The figure shows three views and two pictorial views of one solid part (mm, origin at its lowest corner). Answer the questions. A direction names the side the tool comes from. Coordinates: 2 decimals unless noted, no trailing zeros. Loops run counter-clockwise (first coordinate to the right, second up) from the corner with the lowest first, then second, coordinate; pieces in that order, holes last.
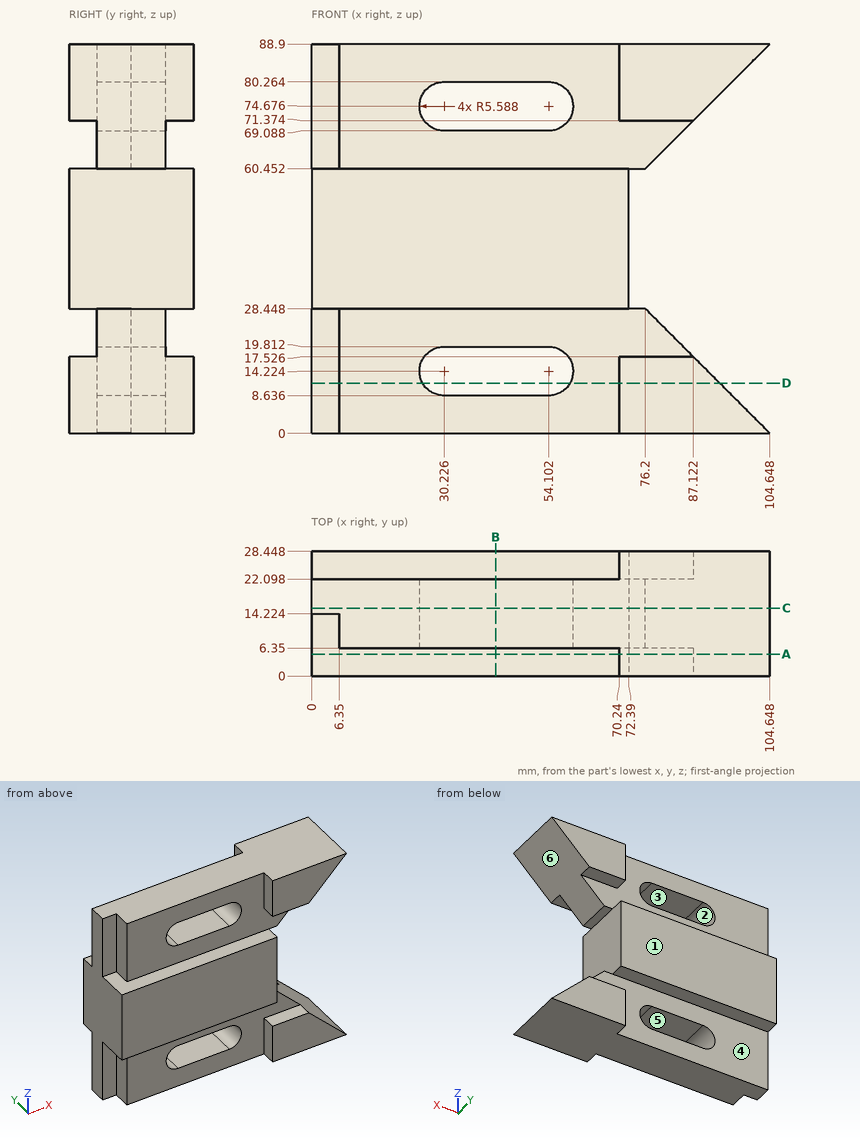
1. A cutting plane is placed at D-D, the plane z = 11.5. Give the vertices of the cut face in (x, y), then the cut area to 3 significant figures.
2. For the marked faces 1 and 2, determine the directions among +Z, -Z, +X, -X, +Y, -Y from which every point of the face is accessible in a straight line to the end or side of a thin tool.
3. A cutting plane is placed at C-C, the plane y = 15.5. Give the vertices of the cut face in (x, z), then the cut area to 3 significant figures.
4. A cutting plane is placed at B-B, the plane x = 42. Give the vertices of the cut face in (y, z), then the cut area to 3 significant figures.
5. Straight lines are drawn through the part: probe 1 along Z at (x, y) = (44.5, 6.75); probe 2 along Z at (x, y) = (78.5, 3.75); probe 3 along Y at (x, z) = (23.5, 19.5). For each, find the intervals that lie inside material, in ascending order.
6. Determine the mould class of the marked faces 3, 4, 5 and 6 for opening direction X: released by +X, released by -X, zero draft, split by the parting line, or undercut.
7. A cutting plane is placed at A-A, the plane y = 5. Give the vertices of the cut face in (x, z).
8. Each of these flat-tipped pins is pushed along its axis until it touches: P1, Ø3, axis at x = 27, y = 26, coming from the -Z side; P2, Ø3, axis at x = 3, z = 75.5, coming from the -Y side; P3, Ø5, axis at x = 23, z = 72, coming from the +Y side; P4, Ø8.5, axis at x = 43.5, z = 15, coming from the +Y side. Where does it stop, or does it pass through?
Answers below:
1. outline: (0, 14.22) - (6.35, 14.22) - (6.35, 6.35) - (25.35, 6.35) - (25.35, 22.1) - (0, 22.1) - close; (58.98, 6.35) - (70.24, 6.35) - (70.24, 0) - (93.15, 0) - (93.15, 28.45) - (70.24, 28.45) - (70.24, 22.1) - (58.98, 22.1) - close
1. area: 1,180 mm2
2. face 1: +Z, -Z, +X, -X, +Y
2. face 2: +Y, -Y
3. outline: (0, 0) - (104.65, 0) - (76.2, 28.45) - (72.39, 28.45) - (72.39, 60.45) - (76.2, 60.45) - (104.65, 88.9) - (0, 88.9) - close; hole (30.23, 8.64) - (54.1, 8.64) arc R5.59 ccw to (54.1, 19.81) - (30.23, 19.81) arc R5.59 ccw to start; hole (30.23, 69.09) - (54.1, 69.09) arc R5.59 ccw to (54.1, 80.26) - (30.23, 80.26) arc R5.59 ccw to start
3. area: 6,730 mm2
4. outline: (0, 28.45) - (6.35, 28.45) - (6.35, 19.81) - (22.1, 19.81) - (22.1, 28.45) - (28.45, 28.45) - (28.45, 60.45) - (22.1, 60.45) - (22.1, 69.09) - (6.35, 69.09) - (6.35, 60.45) - (0, 60.45) - close; (6.35, 0) - (22.1, 0) - (22.1, 8.64) - (6.35, 8.64) - close; (6.35, 80.26) - (22.1, 80.26) - (22.1, 88.9) - (6.35, 88.9) - close
4. area: 1,450 mm2
5. probe 1: z = 0 to 8.64, 19.81 to 69.09, 80.26 to 88.9
5. probe 2: z = 0 to 17.53, 71.37 to 88.9
5. probe 3: y = 6.35 to 22.1
6. face 3: undercut
6. face 4: zero draft
6. face 5: undercut
6. face 6: released by +X
7. outline: (0, 28.45) - (72.39, 28.45) - (72.39, 60.45) - (0, 60.45) - close; (70.24, 0) - (104.65, 0) - (87.12, 17.53) - (70.24, 17.53) - close; (70.24, 71.37) - (87.12, 71.37) - (104.65, 88.9) - (70.24, 88.9) - close
8. P1: stops at z = 28.45
8. P2: stops at y = 14.22
8. P3: stops at y = 22.1
8. P4: passes through
